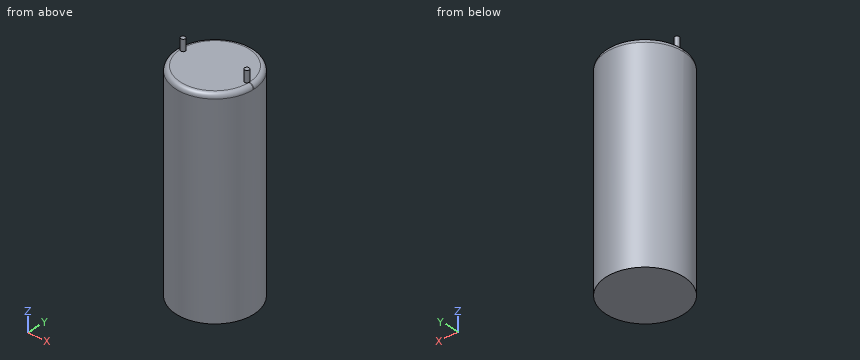
from build123d import *

# Parameters (mm, degrees)
F0_R     = 109.45622
F1_DEPTH = 292.89375
F2_R     = 6.35
F3_DEPTH = 31.75
F4_R     = 12.7


with BuildPart() as f1:
    # F0 (on Top) → F1 (new body, symmetric)
    with BuildSketch(Plane.XY):
        Circle(F0_R)
    extrude(amount=F1_DEPTH, both=True)

    # F2 (on face) → F3 (join)
    with BuildSketch(Plane.XY.offset(292.89375)):
        with Locations((90.4875, 0)):
            Circle(F2_R)
        with Locations((-90.4875, 0)):
            Circle(F2_R)
    extrude(amount=F3_DEPTH)

    # F4
    f4_edges = [f1.edges().sort_by_distance(p)[0] for p in [
        (-109.45622, 0, 292.89375),
    ]]
    fillet(f4_edges, radius=F4_R)


solid = f1.part
Could you check a few things on this model? Use its own coordinates, in mm. Coordinates: 2 decimals unless noted, no trailing zeros. Order: outer loops, then holes, each group sorted by start corner. A loop starts at its lowest first (then second) coordinate and runs counter-clockwise, first axis right, second up. Notation, with made-up numbers: (21, -23.75) - (64, -23.75) arc R27 ccw to (64, 11.25) - close; hole circle Ø7 at (11.25, -39). An arc over 180 degrees is marked (long way). Answer in a Markdown table with one row per item. Add a question column.
(1) If we section it at B-B, the plane z = -180: Please give me the cut outline in (x, y).
(2) Will these pins go through, and if not, where does the flat tip stop? pin 1 (8 mm diameter, centred on x = 61.5, z = 231, fed in from +Y); pin 2 (10 mm diameter, centred on x = -69, z = 127, fed in from -Y); pin 3 (8 mm diameter, centred on y = -79.5, z = 88, fed in from +X).
(3) If we section it at A-A, the plane x = 0: Please give me the cut outline in (y, z), then the cut area to 3 significant figures.
(4) I need wall thicknesses on L1, parallel to Z at x = 46.5, y = 30.5; L2, parallel to Y at x = -4, z = 278.5; L3, parallel to Z at x = -99, y = -27. Which ranges of each line are inside material? Lowest first, please.
Results are:
| question | item | result |
|---|---|---|
| 1 | outline | circle Ø218.91 at (0, 0) |
| 2 | pin 1 | stops at y = 93.14 |
| 2 | pin 2 | stops at y = -88.8 |
| 2 | pin 3 | stops at x = 79.25 |
| 3 | outline | (-109.46, -292.89) - (109.46, -292.89) - (109.46, 280.19) arc R12.7 ccw to (96.76, 292.89) - (-96.76, 292.89) arc R12.7 ccw to (-109.46, 280.19) - close |
| 3 | area | 128,000 mm2 |
| 4 | L1 | z = -292.89 to 292.89 |
| 4 | L2 | y = -109.38 to 109.38 |
| 4 | L3 | z = -292.89 to 291.46 |
